Design review of the part built by this model. Coordinates are the model's own, in mm. A direction names the side the tool comes from. Give positions to 0.01 mm unless a question says otherwise; leave off trailing zeros. Loops run counter-clockwise (first coordinate to the right, second up) from the corner with the lowest first, then second, coordinate; pieces in that order, holes last. Notation, with made-up numbers: (25, -27.75) -> (65, -27.75) arc R22 cw to (65, -11.75) -> close; hole circle Ø10 at (-28, 77). An arc over 180 degrees is marked (long way). Answer as CSV lines item,"result".
from build123d import *

# Parameters (mm, degrees)
SKETCH1_W           = 250.825
SKETCH1_H           = 203.2
SKETCH1_R           = 1.5875
BOSS_EXTRUDE1_DEPTH = 1.5875
SKETCH2_W           = 14.2875
SKETCH2_H           = 139.7
SKETCH2_W_2         = 1.5875
SKETCH2_H_2         = 133.35
SKETCH2_W_3         = 88.9
SKETCH2_H_3         = 9.525
SKETCH2_W_4         = 85.725
SKETCH2_H_4         = 1.5875
BOSS_EXTRUDE2_DEPTH = 6.35
SKETCH3_W           = 23.821163823
SKETCH3_H           = 152.4
BOSS_EXTRUDE3_DEPTH = 33.3375


with BuildPart() as part:
    # Sketch1 → Boss-Extrude1 (new body)
    with BuildSketch(Plane(origin=(0, 0, 0), x_dir=(1, 0, 0), z_dir=(0, 1, 0))):
        with Locations((125.4125, 101.6)):
            Rectangle(SKETCH1_W, SKETCH1_H)
        with Locations(Location((31.75, 196.85, 0), (0, 0, 270))):
            Circle(SKETCH1_R, mode=Mode.SUBTRACT)
        with Locations(Location((165.1, 196.85, 0), (0, 0, 270))):
            Circle(SKETCH1_R, mode=Mode.SUBTRACT)
        with Locations(Location((238.252, 196.85, 0), (0, 0, 270))):
            Circle(SKETCH1_R, mode=Mode.SUBTRACT)
        with Locations(Location((238.252, 38.1, 0), (0, 0, 270))):
            Circle(SKETCH1_R, mode=Mode.SUBTRACT)
        with Locations(Location((190.5, 34.925, 0), (0, 0, 270))):
            Circle(SKETCH1_R, mode=Mode.SUBTRACT)
        with Locations(Location((9.525, 38.1, 0), (0, 0, 270))):
            Circle(SKETCH1_R, mode=Mode.SUBTRACT)
        with Locations(Location((57.15, 166.6875, 0), (0, 0, 270))):
            Circle(SKETCH1_R, mode=Mode.SUBTRACT)
        with Locations(Location((131.7625, 166.6875, 0), (0, 0, 270))):
            Circle(SKETCH1_R, mode=Mode.SUBTRACT)
        with Locations(Location((131.7625, 92.075, 0), (0, 0, 270))):
            Circle(SKETCH1_R, mode=Mode.SUBTRACT)
        with Locations(Location((57.15, 92.075, 0), (0, 0, 270))):
            Circle(SKETCH1_R, mode=Mode.SUBTRACT)
    extrude(amount=BOSS_EXTRUDE1_DEPTH)

    # Sketch2 → Boss-Extrude2 (add)
    # profile 1 of 3: a face of its own
    with BuildSketch(Plane(origin=(0, 1.5875, 0), x_dir=(1, 0, 0), z_dir=(0, 1, 0))):
        with Locations((151.60625, 127)):
            Rectangle(SKETCH2_W, SKETCH2_H)
        with Locations((148.034375, 127)):
            Rectangle(SKETCH2_W_2, SKETCH2_H_2, mode=Mode.SUBTRACT)
        with Locations((155.178125, 127)):
            Rectangle(SKETCH2_W_2, SKETCH2_H_2, mode=Mode.SUBTRACT)
    # profile 2 of 3: a face of its own
    with BuildSketch(Plane(origin=(0, 1.5875, 0), x_dir=(1, 0, 0), z_dir=(0, 1, 0))):
        with Locations((177.00625, 117.475)):
            Rectangle(SKETCH2_W, SKETCH2_H)
        with Locations((173.434375, 117.475)):
            Rectangle(SKETCH2_W_2, SKETCH2_H_2, mode=Mode.SUBTRACT)
        with Locations((180.578125, 117.475)):
            Rectangle(SKETCH2_W_2, SKETCH2_H_2, mode=Mode.SUBTRACT)
    # profile 3 of 3: a face of its own
    with BuildSketch(Plane(origin=(0, 1.5875, 0), x_dir=(1, 0, 0), z_dir=(0, 1, 0))):
        with Locations((87.3125, 20.6375)):
            Rectangle(SKETCH2_W_3, SKETCH2_H_3)
        with Locations((87.3125, 21.43125)):
            Rectangle(SKETCH2_W_4, SKETCH2_H_4, mode=Mode.SUBTRACT)
    extrude(amount=BOSS_EXTRUDE2_DEPTH)

    # Sketch3 → Boss-Extrude3 (add)
    with BuildSketch(Plane(origin=(0, 1.5875, 0), x_dir=(1, 0, 0), z_dir=(0, 1, 0))):
        with Locations((11.910581912, 127)):
            Rectangle(SKETCH3_W, SKETCH3_H)
    extrude(amount=BOSS_EXTRUDE3_DEPTH)


solid = part.part
Q1. We need section C-C, the plane y = 18. State the section outline as (x, z) points.
Filled sheet:
outline,"(0, -203.2) -> (23.82, -203.2) -> (23.82, -50.8) -> (0, -50.8) -> close"
Q2. We need section A-A, the plane x = 110. State the section outline as (y, z) points (1 decimal), and give its area (3 significant figures).
Filled sheet:
outline,"(0, -203.2) -> (1.6, -203.2) -> (1.6, -25.4) -> (7.9, -25.4) -> (7.9, -22.2) -> (1.6, -22.2) -> (1.6, -20.6) -> (7.9, -20.6) -> (7.9, -15.9) -> (1.6, -15.9) -> (1.6, 0) -> (0, 0) -> close"
area,"373 mm^2"
Q3. To check wall thickness, follow probe 1 along Z at (x, y) = (190.5, 0.65); probe 2 along Z at (x, y) = (116, 3) (1 decimal); probe 3 along Y at (x, z) = (139, -181). State the ranges of each line that lie inside material, in increasing order. Write a range as from..to.
Filled sheet:
probe 1,"z = -203.2..-36.51, -33.34..0"
probe 2,"z = -25.4..-22.2, -20.6..-15.9"
probe 3,"y = 0..1.59"
Q4. For faces 1 (the flat face through (144.462, 5, -126)), 2 (the flat face through (152, 5, -196.85)), 3 (the flat face through (87, 5, -15.875)), 4 (the flat face through (174.228, 5, -117)), 5 (the flat face through (152, 5, -57.15)), list the 3-axis set-ups (+Z, -Z, +X, -X, +Y, -Y) from which the entire face can be reached by the end or side of a thin tool; tool diameter is ignored.
Filled sheet:
face 1,"+Z, -Z, +Y"
face 2,"-Z, +X, +Y"
face 3,"+Z, +X, -X, +Y"
face 4,"+Y"
face 5,"+Z, +Y"
Q5. We need section D-D, the plane x = 20. State the section outline as (y, z) points (1 decimal), and give its area (3 significant figures).
Filled sheet:
outline,"(0, -203.2) -> (34.9, -203.2) -> (34.9, -50.8) -> (1.6, -50.8) -> (1.6, 0) -> (0, 0) -> close"
area,"5,400 mm^2"
Q6. Clearance check with flat-ended pins moving along their axes: pin 1 Ø8 at (x, z) = (93.5, -95.5) entering from +Y; pin 2 Ø3 at (x, y) = (153, 5) entering from +Z; pin 3 Ø3 at (x, y) = (92.5, 4) entering from -Z; pin 4 Ø4 at (x, z) = (195.5, -155.5) entering from -Y. State where each tip first meets the part, or that it passes through.
Filled sheet:
pin 1,"stops at y = 1.59"
pin 2,"stops at z = -57.15"
pin 3,"stops at z = -25.4"
pin 4,"stops at y = 0"
